from build123d import *

# Parameters (mm, degrees)
F1_DEPTH = 30
F2_R     = 16
F3_DEPTH = 130
F4_SIZE  = 5
F5_R     = 1


with BuildPart() as f1:
    # F0 (on Top) → F1 (new body)
    with BuildSketch(Plane.XY):
        Polygon((6.831874, -39.832886), (37.912228, -13.999867), (31.080354, 25.83302), (-6.831874, 39.832886), (-37.912228, 13.999867), (-31.080354, -25.83302), align=None)
    extrude(amount=F1_DEPTH)

    # F2 (on face) → F3 (join)
    with BuildSketch(Plane(origin=(0, 0, 0), x_dir=(1, 0, 0), z_dir=(0, 0, -1))):
        Circle(F2_R)
    extrude(amount=F3_DEPTH)

    # F4
    f4_edges = [f1.edges().sort_by_distance(p)[0] for p in [
        (22.372051, -26.916377, 30),
        (-12.12424, -32.832953, 30),
        (-34.496291, -5.916576, 30),
        (-22.372051, 26.916377, 30),
        (12.12424, 32.832953, 30),
        (34.496291, 5.916576, 30),
    ]]
    chamfer(f4_edges, length=F4_SIZE)

    # F5
    f5_edges = [f1.edges().sort_by_distance(p)[0] for p in [
        (6.831874, -39.832886, 12.5),
        (37.912228, -13.999867, 12.5),
        (31.080354, 25.83302, 12.5),
        (-6.831874, 39.832886, 12.5),
        (-37.912228, 13.999867, 12.5),
        (-31.080354, -25.83302, 12.5),
    ]]
    fillet(f5_edges, radius=F5_R)


solid = f1.part
Work out the finished part from the listing and answer in its coordinate system (mm). A direction names the side the tool comes from. Round coordinates to 2 decimals unless told otherwise and drop trailing zeros. Loops run counter-clockwise (first coordinate to the right, second up) from the corner with the lowest first, then second, coordinate; pieces in that order, holes last. Notation, with made-up numbers: M -14.5,-31 L 7.5,-31 A18 cw 7.5,1 Z; hole C 51.25,81.25 d2. An arc over 180 degrees is marked long. One line per question, with ' | ' between items. Start each with the question number.
(1) Flat-ended cylindrical pins translate along their axes: pin 1 Ø1 at (x, y) = (-14, -20.5) entering from -Z; pin 2 Ø10 at (x, z) = (-0.5, -9) entering from -Y; pin 3 Ø1.5 at (x, z) = (17.5, -56) entering from -Y; pin 4 Ø4 at (x, z) = (16, -44.5) entering from -Y. Find the tip coordinate at first contact, or state that the pin passes through.
(2) A cutting plane is placed at A-A on x = 0. Write down the section's boundary in (y, z).
(3) A tool of negligible diameter and unlimited length cuts with its end or side. For faces 1 (the face through (0, 0, 30)), 2 (the face through (-3.47, 15.62, -64.09)), from which of +Z, -Z, +X, -X, +Y, -Y can it reach the whole face along a straight path? Write none if from no direction.
(4) A cutting plane is placed at D-D on x = 23. Write down the section's boundary in (y, z).
(5) A cutting plane is placed at C-C on y = 0. Write down the section's boundary in (x, z), plus the area to 3 significant figures.
(6) Find the intervals of material crossed by line 1 (Z direction, x = 2.5, y = -23.5); line 2 (X direction, y = -0.5, z = -53); line 3 (X direction, y = 2, z = -97), in increasing order.
(7) A cutting plane is placed at B-B on z = -85. Write down the section's boundary in (x, y), plus the area to 3 significant figures.
Geometry check:
1) pin 1: stops at z = 0 | pin 2: stops at y = -16 | pin 3: passes through | pin 4: stops at y = -7.75
2) outline: M -37.31,0 L -16,0 L -16,-130 L 16,-130 L 16,0 L 37.31,0 L 37.31,25 L 31.98,30 L -31.98,30 L -37.31,25 Z
3) face 1: +Z, +X, -X, +Y, -Y | face 2: -Z
4) outline: M -26.39,0 L 28.82,0 L 28.82,25 L 23.49,30 L -19.89,30 L -26.39,25 Z
5) outline: M -35.51,0 L -16,0 L -16,-130 L 16,-130 L 16,0 L 35.51,0 L 35.51,25 L 30.44,30 L -30.44,30 L -35.51,25 Z | area: 6,270 mm²
6) line 1: z = 0 to 30 | line 2: x = -15.99 to 15.99 | line 3: x = -15.87 to 15.87
7) outline: C 0,0 d32 | area: 804 mm²
